from build123d import *

# Parameters (mm, degrees)
ESQUISSE1_W             = 86
ESQUISSE1_H             = 185
BOSS_EXTRU_1_DEPTH      = 9
ESQUISSE2_R             = 1.65
ENL_V_MAT_EXTRU_1_DEPTH = 205.210675529
ESQUISSE3_R             = 1.65
ENL_V_MAT_EXTRU_2_DEPTH = 205.210675529
ESQUISSE4_W             = 4
ESQUISSE4_H             = 32
ENL_V_MAT_EXTRU_3_DEPTH = 205.210675529
ENL_V_MAT_EXTRU_4_DEPTH = 205.210675529
ESQUISSE7_W             = 12
ESQUISSE7_H             = 10
ENL_V_MAT_EXTRU_5_DEPTH = 205.210675529
CONG_1_R                = 4


with BuildPart() as part:
    # Esquisse1 → Boss.-Extru.1 (new body)
    with BuildSketch(Plane.XY):
        with Locations((43, 92.5)):
            Rectangle(ESQUISSE1_W, ESQUISSE1_H)
    extrude(amount=BOSS_EXTRU_1_DEPTH)

    # Esquisse2 → Enlèv. mat.-Extru.1 (cut, through all)
    with BuildSketch(Plane.XY.offset(9)):
        with Locations((8, 57.5)):
            Circle(ESQUISSE2_R)
        with Locations(Location((28, 57.5, 0), (0, 0, 180))):
            Circle(ESQUISSE2_R)
        with Locations((28, 37.5)):
            Circle(ESQUISSE2_R)
        with Locations(Location((8, 37.5, 0), (0, 0, 180))):
            Circle(ESQUISSE2_R)
        with Locations((78, 37.5)):
            Circle(ESQUISSE2_R)
        with Locations(Location((58, 37.5, 0), (0, 0, 180))):
            Circle(ESQUISSE2_R)
        with Locations((58, 57.5)):
            Circle(ESQUISSE2_R)
        with Locations(Location((78, 57.5, 0), (0, 0, 180))):
            Circle(ESQUISSE2_R)
        with Locations((78, 97.5)):
            Circle(ESQUISSE2_R)
        with Locations(Location((58, 97.5, 0), (0, 0, 180))):
            Circle(ESQUISSE2_R)
        with Locations((58, 117.5)):
            Circle(ESQUISSE2_R)
        with Locations(Location((78, 117.5, 0), (0, 0, 180))):
            Circle(ESQUISSE2_R)
        with Locations((8, 117.5)):
            Circle(ESQUISSE2_R)
        with Locations(Location((28, 117.5, 0), (0, 0, 180))):
            Circle(ESQUISSE2_R)
        with Locations((28, 97.5)):
            Circle(ESQUISSE2_R)
        with Locations(Location((8, 97.5, 0), (0, 0, 180))):
            Circle(ESQUISSE2_R)
    extrude(amount=-ENL_V_MAT_EXTRU_1_DEPTH, mode=Mode.SUBTRACT)

    # Esquisse3 → Enlèv. mat.-Extru.2 (cut, through all)
    with BuildSketch(Plane.XY.offset(9)):
        with Locations((8, 28)):
            Circle(ESQUISSE3_R)
        with Locations(Location((8, 8, 0), (0, 0, 180))):
            Circle(ESQUISSE3_R)
        with Locations((28, 8)):
            Circle(ESQUISSE3_R)
        with Locations(Location((28, 28, 0), (0, 0, 180))):
            Circle(ESQUISSE3_R)
        with Locations((28, 68)):
            Circle(ESQUISSE3_R)
        with Locations(Location((28, 88, 0), (0, 0, 180))):
            Circle(ESQUISSE3_R)
        with Locations((8, 88)):
            Circle(ESQUISSE3_R)
        with Locations(Location((8, 68, 0), (0, 0, 180))):
            Circle(ESQUISSE3_R)
        with Locations((78, 68)):
            Circle(ESQUISSE3_R)
        with Locations(Location((78, 88, 0), (0, 0, 180))):
            Circle(ESQUISSE3_R)
        with Locations((58, 88)):
            Circle(ESQUISSE3_R)
        with Locations(Location((58, 68, 0), (0, 0, 180))):
            Circle(ESQUISSE3_R)
        with Locations((58, 28)):
            Circle(ESQUISSE3_R)
        with Locations(Location((58, 8, 0), (0, 0, 180))):
            Circle(ESQUISSE3_R)
        with Locations((78, 8)):
            Circle(ESQUISSE3_R)
        with Locations(Location((78, 28, 0), (0, 0, 180))):
            Circle(ESQUISSE3_R)
    extrude(amount=-ENL_V_MAT_EXTRU_2_DEPTH, mode=Mode.SUBTRACT)

    # Esquisse4 → Enlèv. mat.-Extru.3 (cut, through all)
    with BuildSketch(Plane.XY.offset(9)):
        with Locations((2, 16)):
            Rectangle(ESQUISSE4_W, ESQUISSE4_H)
        with Locations((84, 16)):
            Rectangle(ESQUISSE4_W, ESQUISSE4_H)
    extrude(amount=-ENL_V_MAT_EXTRU_3_DEPTH, mode=Mode.SUBTRACT)

    # Esquisse6 → Enlèv. mat.-Extru.4 (cut, through all)
    with BuildSketch(Plane.XY.offset(9)):
        with BuildLine():
            Line((22, 167), (32, 167))
            ThreePointArc((32, 167), (34, 165), (32, 163))
            Line((32, 163), (22, 163))
            ThreePointArc((22, 163), (20, 165), (22, 167))
        make_face()
        with BuildLine():
            Line((22, 139), (32, 139))
            ThreePointArc((32, 139), (34, 141), (32, 143))
            Line((32, 143), (22, 143))
            ThreePointArc((22, 143), (20, 141), (22, 139))
        make_face()
        with BuildLine():
            Line((74, 167), (64, 167))
            ThreePointArc((64, 167), (62, 165), (64, 163))
            Line((64, 163), (74, 163))
            ThreePointArc((74, 163), (76, 165), (74, 167))
        make_face()
        with BuildLine():
            Line((74, 139), (64, 139))
            ThreePointArc((64, 139), (62, 141), (64, 143))
            Line((64, 143), (74, 143))
            ThreePointArc((74, 143), (76, 141), (74, 139))
        make_face()
    extrude(amount=-ENL_V_MAT_EXTRU_4_DEPTH, mode=Mode.SUBTRACT)

    # Esquisse7 → Enlèv. mat.-Extru.5 (cut, through all)
    with BuildSketch(Plane.XY.offset(9)):
        with Locations((43, 180)):
            Rectangle(ESQUISSE7_W, ESQUISSE7_H)
    extrude(amount=-ENL_V_MAT_EXTRU_5_DEPTH, mode=Mode.SUBTRACT)

    # Congé1
    cong_1_edges = [part.edges().sort_by_distance(p)[0] for p in [
        (0, 185, 4.5),
        (86, 185, 4.5),
    ]]
    fillet(cong_1_edges, radius=CONG_1_R)


solid = part.part
Check sheet for the modelled part. Datum: model origin and axes. Units: mm. A direction names the side the tool comes from. Coordinates: 2 decimals unless noted, no trailing zeros. Write each loop counter-clockwise with the first axis right and the second up, starting at its lowest first coordinate (ties: lowest second). Pieces come first, ordered by that corner, then holes.
Item 1: Cross-section at A-A on y = 37.5. Record the boundary of the cut face in (x, z), then the cut area to 3 significant figures.
Numbers:
outline: (0, 0) - (6.35, 0) - (6.35, 9) - (0, 9) - close; (9.65, 0) - (26.35, 0) - (26.35, 9) - (9.65, 9) - close; (29.65, 0) - (56.35, 0) - (56.35, 9) - (29.65, 9) - close; (59.65, 0) - (76.35, 0) - (76.35, 9) - (59.65, 9) - close; (79.65, 0) - (86, 0) - (86, 9) - (79.65, 9) - close
area: 655 mm2
Item 2: Cross-section at C-C on y = 141. Record the boundary of the cut face in (x, z), then the cut area to 3 significant figures.
Numbers:
outline: (0, 0) - (20, 0) - (20, 9) - (0, 9) - close; (34, 0) - (62, 0) - (62, 9) - (34, 9) - close; (76, 0) - (86, 0) - (86, 9) - (76, 9) - close
area: 522 mm2
Item 3: Cross-section at B-B on x = 66. Record the boundary of the cut face in (y, z).
Numbers:
outline: (0, 0) - (139, 0) - (139, 9) - (0, 9) - close; (143, 0) - (163, 0) - (163, 9) - (143, 9) - close; (167, 0) - (185, 0) - (185, 9) - (167, 9) - close
Item 4: Cross-section at D-D on z = 4.5. Count the separate pieces of the cut face and the enclosed holes in it, then the cut area to 3 significant figures.
Numbers:
separate pieces: 1
enclosed holes: 36
area: 15,000 mm2
Item 5: Depth check by flat-ended pin: pin 1 Ø2.5 at (x, y) = (28, 88) entering from +Z; pin 2 Ø4.5 at (y, z) = (20, 4.5) entering from -X; pin 3 Ø3 at (x, z) = (85, 2.5) entering from -Y. Enter the tip coordinate at first touch or a pass-through.
Numbers:
pin 1: passes through
pin 2: stops at x = 4
pin 3: stops at y = 32
Item 6: Mould release check, pull along Y, two halves, no side actions. Record for faces 1 (the face through (43, 175, 5)), 2 (the face through (0, 105, 4)), 3 (the face through (62, 165, 5)): released by +Y, released by -Y, zero draft, split by the parting line, or undercut.
Numbers:
face 1: released by +Y
face 2: zero draft
face 3: undercut
Item 7: Access from +Z, -Z, +X, -X, +Y, -Y to the whole of each face (thin tool, end or side, straight path). Record for faces 4 (the face through (4, 16, 5)), 5 (the face through (82, 16, 5)), 6 (the face through (34, 165, 5)).
Numbers:
face 4: +Z, -Z, -X, -Y
face 5: +Z, -Z, +X, -Y
face 6: +Z, -Z
Item 8: Scan lines: probe 1 along Y at (x, z) = (66.5, 3); probe 2 along X at (y, z) = (88, 5.5); probe 3 along X at (y, z) = (177.5, 8.5). Record each from-to range of solid material in increasing order.
Numbers:
probe 1: y = 0 to 139, 143 to 163, 167 to 185
probe 2: x = 0 to 6.35, 9.65 to 26.35, 29.65 to 56.35, 59.65 to 76.35, 79.65 to 86
probe 3: x = 0 to 37, 49 to 86
